Source: CAD feature listing. Evaluate the final solid. Frame: model axes, mm. A direction names the side the tool comes from. Round coordinates to 2 decimals unless told otherwise and drop trailing zeros. Write each loop counter-clockwise with the first axis right and the second up, starting at its lowest first coordinate (ties: lowest second). Pieces come first, ordered by that corner, then holes. Notation, with made-up numbers: (65.25, -23.5) -> (98.25, -23.5) arc R20 ccw to (98.25, -5.5) -> close; hole circle Ø3 at (-11.75, 87). An arc over 180 degrees is marked (long way). Put each result on its own line as item: value.
```python
from build123d import *

# Parameters (mm, degrees)
SKETCH4_W           = 80
SKETCH4_H           = 50
BOSS_EXTRUDE2_DEPTH = 7
CUT_EXTRUDE2_DEPTH  = 4


with BuildPart() as part:
    # Sketch4 → Boss-Extrude2 (new body)
    with BuildSketch(Plane.XY):
        Rectangle(SKETCH4_W, SKETCH4_H)
    extrude(amount=-BOSS_EXTRUDE2_DEPTH)

    # Sketch8 → Cut-Extrude2 (cut)
    with BuildSketch(Plane(origin=(0, 0, -7), x_dir=(-1, 0, 0), z_dir=(0, 0, -1))):
        with BuildLine():
            Line((-30, 4), (30, 4))
            ThreePointArc((30, 4), (34, 0), (30, -4))
            Line((30, -4), (-30, -4))
            ThreePointArc((-30, -4), (-34, 0), (-30, 4))
        make_face()
    extrude(amount=-CUT_EXTRUDE2_DEPTH, mode=Mode.SUBTRACT)


solid = part.part
```
Q1. Reachability of faces 4 (the flat face through (-1, 6, -7)), 5 (the flat face through (0, 4, -5)) from +Z, -Z, +X, -X, +Y, -Y: full face, straight path, thin tool, end or side. Return the list, or none.
Ans:
face 4: -Z, +X, -X, +Y, -Y
face 5: -Z
Q2. Material intervals for line 1 (Y direction, x = 18, z = -6.5); line 2 (Z direction, x = -23, y = 0); line 3 (Y direction, x = 32, z = -4.25), sorted ascending. Write a range as [from, to].
Ans:
line 1: y = [-25, -4], [4, 25]
line 2: z = [-3, 0]
line 3: y = [-25, -3.46], [3.46, 25]
Q3. Cut plane B-B on y = 0. Output: boundary loops of the cut face in (x, z), and give its area (3 significant figures).
Ans:
outline: (-40, -7) -> (-34, -7) -> (-34, -3) -> (34, -3) -> (34, -7) -> (40, -7) -> (40, 0) -> (-40, 0) -> close
area: 288 mm^2
Q4. Cut plane C-C on x = -21.5. Output: boundary loops of the cut face in (y, z).
Ans:
outline: (-25, -7) -> (-4, -7) -> (-4, -3) -> (4, -3) -> (4, -7) -> (25, -7) -> (25, 0) -> (-25, 0) -> close
Q5. Draft query along X for faces 1 (the flat face through (0, -4, -5)), 2 (the flat face through (-1, -25, -3)), 3 (the flat face through (40, 0, -3)). Return one class per face: +X half, -X half, draft (parallel to the pull), parting line (faces both ways), or undercut.
Ans:
face 1: undercut
face 2: draft
face 3: +X half
Q6. Pin query (flat end, axial travel): pin 1 (10 mm diameter, centred on x = -15, y = -13, fed in from +Z); pin 2 (6.5 mm diameter, centred on x = 4.5, y = 0.5, fed in from -Z). Return the tip coordinate at first contact, or that it passes through.
Ans:
pin 1: stops at z = 0
pin 2: stops at z = -3
Q7. Cut plane A-A on z = -4.5. Output: boundary loops of the cut face in (x, y).
Ans:
outline: (-40, -25) -> (40, -25) -> (40, 25) -> (-40, 25) -> close; hole (-30, -4) -> (30, -4) arc R4 ccw to (30, 4) -> (-30, 4) arc R4 ccw to start
